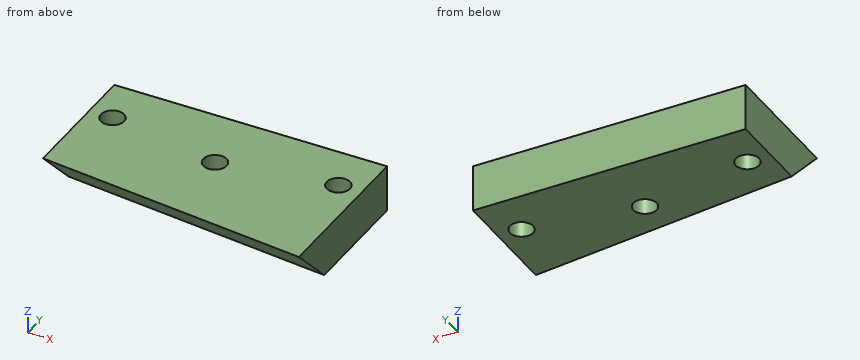
```python
from build123d import *

# Parameters (mm, degrees)
F1_DEPTH = 6
F2_SIZE  = 5.99999
F3_R     = 1.5
F4_DEPTH = 6


# Not quite as in the source:
# - a fillet or chamfer is up to 0.001 mm smaller than in the source, because OpenCascade refuses the exact size


with BuildPart() as f1:
    # F0 (on Top) → F1 (new body)
    with BuildSketch(Plane.XY):
        Polygon((31.2662842423, 6.9127185345), (-3.7337157577, 6.9127185345), (-3.7337157577, -10.0872814655), (31.2662842423, -14.0872814655), align=None)
    extrude(amount=F1_DEPTH)

    # F2 (size 6 in the source; OpenCascade refuses exactly that, so slightly less here)
    f2_edges = [f1.edges().sort_by_distance(p)[0] for p in [
        (13.766284, -12.087281, 0),
    ]]
    chamfer(f2_edges, length=F2_SIZE)

    # F3 (on face) → F4 (cut, through all)
    with BuildSketch(Plane.XY.offset(6)):
        with Locations((-0.7337157577, 0.9127185345)):
            Circle(F3_R)
        with Locations((13.7662842423, -1.5872814655)):
            Circle(F3_R)
        with Locations((28.2662842423, 0.9127185345)):
            Circle(F3_R)
    extrude(amount=-F4_DEPTH, mode=Mode.SUBTRACT)


solid = f1.part
```
The listing builds one solid part. Answer for the finished solid, in the listing's coordinates (mm). Give positions to 0.01 mm unless a question says otherwise; leave off trailing zeros. Order: outer loops, then holes, each group sorted by start corner. A loop starts at its lowest first (then second) coordinate and runs counter-clockwise, first axis right, second up.
1) Find section D-D on z = 5.5. Write down the section's boundary in (x, y).
Reported:
outline: (-3.73, -9.58) - (31.27, -13.58) - (31.27, 6.91) - (-3.73, 6.91) - close; hole circle Ø3 at (-0.73, 0.91); hole circle Ø3 at (13.77, -1.59); hole circle Ø3 at (28.27, 0.91)
2) Find section B-B on z = 1.5. Write down the section's boundary in (x, y), then the cut area to 3 significant figures.
Reported:
outline: (-3.73, -5.56) - (31.27, -9.56) - (31.27, 6.91) - (-3.73, 6.91) - close; hole circle Ø3 at (-0.73, 0.91); hole circle Ø3 at (13.77, -1.59); hole circle Ø3 at (28.27, 0.91)
area: 485 mm2
3) Consider line 1 along X through (y, z) = (-1.5, 2.25); line 2 along X through (y, z) = (-2.25, 4); line 3 along Y through (x, z) = (0, 5.75). Determine where each line is inside the solid, lowest interval first.
Reported:
line 1: x = -3.73 to 12.27, 15.26 to 31.27
line 2: x = -3.73 to 12.42, 15.11 to 31.27
line 3: y = -10.26 to -0.4, 2.22 to 6.91
4) Given P1, Ø1, axis at x = 3, z = 1, coming from the -Y side, flat-ended and moving along its own axis, determine where the tip first touches the part or whether it passes through.
Reported:
P1: stops at y = -6.33
